Could you check a few things on this model? Use its own coordinates, in mm. A direction names the side the tool comes from. Give positions to 0.01 mm unless a question says otherwise; leave off trailing zeros. Loops run counter-clockwise (first coordinate to the right, second up) from the corner with the lowest first, then second, coordinate; pieces in that order, holes last. Notation, with made-up numbers: (84, -23) -> (140, -23) arc R15 cw to (140, 6) -> close; hole circle Ø4 at (-3, 25). An arc over 180 degrees is marked (long way). Write item = value, one per line. Start each with the question number.
1) I want a section at B-B (z = -3). List the corners of the cut face in (x, y) for me, and give its area (3 significant figures).
2) I'm going to push flat-ended pins straight in: pin 1 Ø1 at (y, z) = (2, 11.5) entering from +X; pin 2 Ø3.5 at (x, z) = (0, -6) entering from +Y; pin 3 Ø0.5 at (x, y) = (-0.5, -0.5) entering from -Z. Where does each tip first touch, or does it pass through?
3) If we mould it in two halves opening along X, with no side actions, what happens to faces 4 (the face through (0, 1, -18)), 5 (the face through (1, 1, 1)), 6 (the face through (0, 0, 10))? For each: +X half, -X half, draft (parallel to the pull), parting line (faces both ways), or undercut.
4) I want a section at C-C (y = 1.55). List the corners of the cut face in (x, z) for me.
5) I want a section at A-A (x = 0). List the corners of the cut face in (y, z) for me.
6) I need wall thicknesses on probe 1 along Z at (x, y) = (0, -0.5); probe 2 along X at (y, z) = (-0.4, 0); probe 3 along Y at (x, z) = (1.25, -10). Which ranges of each line are inside material? Lowest first, please. Write a range as from..to.
7) I want a section at D-D (z = 6). List the corners of the cut face in (x, y) for me, and give its area (3 significant figures).
8) On a 3-axis mill with a long thin cutter (end or side, diameter ignored), from which of +Z, -Z, +X, -X, +Y, -Y can I reach the whole of each face in a straight line? I mean faces 1 (the face through (0, -0.5, -5)), 2 (the face through (-0.54, 2.48, -2.44)), 3 (the face through (0, -0.5, 5)). Say none if no direction works.
Autodesk Inventor part; units mm, degrees
ref_plane "YZ Plane" through (0, 0, 0) normal (1, 0, 0) x (0, 1, 0)
ref_plane "XZ Plane" through (0, 0, 0) normal (0, 1, 0) x (-1, 0, 0)
ref_plane "XY Plane" through (0, 0, 0) normal (0, 0, 1) x (1, 0, 0)
sketch "Sketch1" plane through (0, 0, 0) normal (0, 1, 0) x (-1, 0, 0)
  circle A0 centre (0, 0) radius 3.7
  circle A1 centre (0, 16) radius 2
  line L0 (0, 16) -> (0, 0) construction
  line L1 (1.9887, 16.2125) -> (3.6791, 0.3931)
  line L2 (-3.6791, 0.3931) -> (-1.9887, 16.2125)
  line L3 (0, 16) -> (0, 18) construction
  line L4 (0, 0) -> (3.7, 0) construction
  circle A2 centre (0, -16) radius 2
  line L5 (0, -16) -> (0, 0) construction
  line L6 (1.9887, -16.2125) -> (3.6791, -0.3931)
  line L7 (-3.6791, -0.3931) -> (-1.9887, -16.2125)
  line L8 (0, -16) -> (0, -18) construction
  point P0 (3.6791, -0.3931)
  dimension "d0" = 4
  dimension "d1" = 7.4
  dimension "d2" = 18
extrude "Extrusion1" add sketch "Sketch1" along normal blind 2
sketch "Sketch2" plane through (0, 2, 0) normal (0, 1, 0) x (1, 0, 0)
  circle A0 centre (0, 0) radius 3.7
  arc A1 (3.6791, -0.3931) -> (3.6791, 0.3931) centre (0, 0) ccw
  line L0 (3.6791, 0.3931) -> (1.9887, 16.2125)
  arc A2 (1.9887, 16.2125) -> (-1.9887, 16.2125) centre (0, 16) ccw
  line L1 (-1.9887, 16.2125) -> (-3.6791, 0.3931)
  arc A3 (-3.6791, 0.3931) -> (-3.6791, -0.3931) centre (0, 0) ccw
  line L2 (-3.6791, -0.3931) -> (-1.9887, -16.2125)
  arc A4 (-1.9887, -16.2125) -> (1.9887, -16.2125) centre (0, -16) ccw
  line L3 (1.9887, -16.2125) -> (3.6791, -0.3931)
  circle A5 centre (0, 0) radius 2.5
  point P0 (-3.7, 0)
  dimension "d5" = 1.2
extrude "Extrusion2" add sketch "Sketch2" along normal blind 2 contours A0
extrude "Extrusion3" cut sketch "Sketch2" against normal blind 1 contours A5
sketch "Sketch3" plane through (0, 0, 0) normal (0, -1, 0) x (1, 0, 0)
  arc A0 (3.6791, -0.3931) -> (3.6791, 0.3931) centre (0, 0) ccw
  line L0 (1.9887, 16.2125) -> (3.6791, 0.3931)
  arc A1 (1.9887, 16.2125) -> (-1.9887, 16.2125) centre (0, 16) ccw
  line L1 (-3.6791, 0.3931) -> (-1.9887, 16.2125)
  arc A2 (-3.6791, 0.3931) -> (-3.6791, -0.3931) centre (0, 0) ccw
  line L2 (-1.9887, -16.2125) -> (-3.6791, -0.3931)
  arc A3 (-1.9887, -16.2125) -> (1.9887, -16.2125) centre (0, -16) ccw
  line L3 (3.6791, -0.3931) -> (1.9887, -16.2125)
  line L4 (3.1868, 5) -> (-3.1868, 5)
  line L5 (3.1868, -5) -> (-3.1868, -5)
  line L6 (0, 5) -> (0, -5) construction
  dimension "d10" = 10
extrude "Extrusion4" add sketch "Sketch3" along normal blind 1 contours L3 L5 L2 A2 L1 L4 L0 A0
sketch "Sketch4" plane through (0, 1, 0) normal (0, 1, 0) x (1, 0, 0)
  point P0 (0, 0)
  point P1 (0, 0)
hole "Hole1" at (0, 1, 0) direction (0, -1, 0) diameter 2.3 end through all
properties part number "MG90s Arm"
Answer list:
q1.outline = (-3.4, -1) -> (3.4, -1) -> (3.4, 2) -> (2.17, 2) -> (2.17, 4) -> (-2.17, 4) -> (-2.17, 2) -> (-3.4, 2) -> close
q1.area = 29.1 mm^2
q2.pin_1 = 2.55
q2.pin_2 = 2
q2.pin_3 = -5
q3.face_4 = parting line
q3.face_5 = undercut
q3.face_6 = draft
q4.outline = (-3.68, -0.39) -> (-1.99, -16.21) arc R2 ccw to (1.99, -16.21) -> (3.68, -0.39) arc R3.7 ccw to (3.68, 0.39) -> (1.99, 16.21) arc R2 ccw to (-1.99, 16.21) -> (-3.68, 0.39) arc R3.7 ccw to start; hole circle Ø5 at (0, 0)
q5.outline = (-1, -5) -> (0, -5) -> (0, -18) -> (2, -18) -> (2, -3.7) -> (4, -3.7) -> (4, -2.5) -> (1, -2.5) -> (1, -1.15) -> (-1, -1.15) -> close; (-1, 1.15) -> (1, 1.15) -> (1, 2.5) -> (4, 2.5) -> (4, 3.7) -> (2, 3.7) -> (2, 18) -> (0, 18) -> (0, 5) -> (-1, 5) -> close
q6.probe_1 = -5..-1.15, 1.15..5
q6.probe_2 = -3.7..-1.15, 1.15..3.7
q6.probe_3 = 0..2
q7.outline = (-3.08, 0) -> (3.08, 0) -> (3.08, 2) -> (-3.08, 2) -> close
q7.area = 12.3 mm^2
q8.face_1 = -Z, +X, -X, -Y
q8.face_2 = +Y
q8.face_3 = +Z, +X, -X, -Y
